Autodesk Inventor part; units mm, degrees
ref_plane "YZ Plane" through (0, 0, 0) normal (1, 0, 0) x (0, 1, 0)
ref_plane "XZ Plane" through (0, 0, 0) normal (0, 1, 0) x (-1, 0, 0)
ref_plane "XY Plane" through (0, 0, 0) normal (0, 0, 1) x (1, 0, 0)
sketch "Эскиз1" plane through (0, 0, 0) normal (0, 1, 0) x (-1, 0, 0)
  line L0 (0, 0) -> (17.5, 0)
  line L1 (17.5, 0) -> (17.5, -16)
  line L2 (17.5, -16) -> (0, -16)
  line L3 (0, -16) -> (0, 0)
  dimension "d0" = 17.5
  dimension "d1" = 16
extrude "Выдавливание1" add sketch "Эскиз1" along normal blind 7.5
sketch "Эскиз2" plane through (0, 7.5, 0) normal (0, 1, 0) x (1, 0, 0)
  line L0 (-17.5, 16) -> (-17.5, 0)
  line L1 (-17.5, 8) -> (-12.5, 8)
  circle A0 centre (-12.5, 8) radius 4
  point P0 (0, 0)
  dimension "d4" = 5
  dimension "d5" = 8
extrude "Выдавливание2" cut sketch "Эскиз2" against normal blind 3
fillet "Сопряжение1" radius 8 2 edges at (-17.5, 3.75, 0) (-17.5, 3.75, -16)
sketch "Эскиз3" plane through (0, 0, 0) normal (0, -1, 0) x (1, 0, 0)
  line L0 (0, 0) -> (0, -16)
  line L1 (0, -8) -> (-2.5, -8)
  line L2 (-2.5, -3.5) -> (-2.5, -12.5)
  dimension "d9" = 2.5
  dimension "d10" = 9
hole "Отверстие1" at (-2.5, 0, -3.5) at (-2.5, 0, -12.5) direction (0, 1, 0) diameter 2.2 end through all countersink diameter 4.5 countersink angle 90
sketch "Эскиз4" plane through (0, 7.5, 0) normal (0, 1, 0) x (1, 0, 0)
  line L0 (0, 0) -> (-5, 0)
  line L1 (-5, 0) -> (-5, 16)
  line L2 (-5, 16) -> (0, 16)
  line L3 (0, 16) -> (0, 0)
  line L4 (0, 16) -> (-9.5, 16)
  dimension "d18" = 5
extrude "Выдавливание3" cut sketch "Эскиз4" against normal blind 3.5
properties part number "Деталь основы рулевого управления"
Read the model definition and answer for the solid it produces. Units are mm, in the model's axes. A direction names the side the tool comes from. Give positions to 0.01 mm unless a question says otherwise; leave off trailing zeros. Loops run counter-clockwise (first coordinate to the right, second up) from the corner with the lowest first, then second, coordinate; pieces in that order, holes last. Notation, with made-up numbers: M 60.5,12 L 115.5,12 A5 ccw 115.5,17 Z; hole C 74,19 d1. An arc over 180 degrees is marked long. Write each question's results on one line, items separated by ' | '.
1. Section A-A on x = -2.5 is taken. Give the vertices of the cut face in (y, z).
Values:
outline: M 0,-16 L 4,-16 L 4,-13.6 L 1.15,-13.6 L 0,-14.75 Z; M 0,-10.25 L 1.15,-11.4 L 4,-11.4 L 4,-4.6 L 1.15,-4.6 L 0,-5.75 Z; M 0,-1.25 L 1.15,-2.4 L 4,-2.4 L 4,0 L 0,0 Z
2. Given pin 1 (3 mm diameter, centred on y = 6, z = -9, fed in from +X); pin 2 (3.5 mm diameter, centred on x = -2.5, z = -3.5, fed in from -Y); pin 3 (1.5 mm diameter, centred on x = -3, z = -7.5, fed in from +Y), each flat-ended and moving along its own axis, determine where each tip first touches the part or whether it passes through.
Values:
pin 1: stops at x = -5 | pin 2: stops at y = 0.5 | pin 3: stops at y = 4
3. The mould has two halves that part along Z. Classify faces 1 (the face through (-15.094, 3.802, -13.719)), 2 (the face through (-13, 4.5, -8)), 3 (the face through (-9, 0, -8)): pulls with the +Z half, pulls with the -Z half, needs draft (parallel to the pull), parting line crosses it, or undercut.
Values:
face 1: pulls with the -Z half | face 2: undercut | face 3: needs draft
4. A tool of negligible diameter and unlimited length cuts with its end or side. For faces 4 (the face through (-5, 6, -8)), 5 (the face through (-13.367, 6.021, -4.095)), 6 (the face through (-2.079, 2.595, -4.516)), from which of +Z, -Z, +X, -X, +Y, -Y can it reach the whole face along a straight path? Write none if from no direction.
Values:
face 4: +Z, -Z, +X, +Y | face 5: +Y | face 6: +Y, -Y
5. Section D-D on z = -3.5 is taken. Give the vertices of the cut face in (x, y), plus the area to 3 significant figures.
Values:
outline: M -16.11,0 L -4.75,0 L -3.6,1.15 L -3.6,4 L -5,4 L -5,7.5 L -16.11,7.5 Z; M -1.4,1.15 L -0.25,0 L 0,0 L 0,4 L -1.4,4 Z | area: 93.2 mm^2
6. Section C-C on y = 3.75 is taken. State how many separate pieces and enclosed holes the cut face has, plus the area to 3 significant figures.
Values:
separate pieces: 1 | enclosed holes: 2 | area: 245 mm^2
7. Straight lines are drawn through the part: line 1 (Z direction, x = -2.5, y = 3.3); line 2 (Y direction, x = -1, z = -7.25); line 3 (X direction, y = 4.75, z = -9.25). For each, find the intervals that lie inside material, in ascending order. Write a range as [from, to].
Values:
line 1: z = [-16, -13.6], [-11.4, -4.6], [-2.4, 0] | line 2: y = [0, 4] | line 3: x = [-17.4, -16.3], [-8.7, -5]
